Could you check a few things on this model? Use its own coordinates, in mm. A direction names the side the tool comes from. Give positions to 0.01 mm unless a question says otherwise; leave off trailing zeros. One line per item, written item: value.
Autodesk Inventor part; units mm, degrees
ref_plane "YZ Plane" through (0, 0, 0) normal (1, 0, 0) x (0, 1, 0)
ref_plane "XZ Plane" through (0, 0, 0) normal (0, 1, 0) x (-1, 0, 0)
ref_plane "XY Plane" through (0, 0, 0) normal (0, 0, 1) x (1, 0, 0)
sketch "Sketch1" plane through (0, 0, 0) normal (0, 1, 0) x (1, 0, 0)
  line L0 (300, 0) -> (-300, 0)
  line L1 (-300, 0) -> (-300, -600)
  line L2 (-300, -600) -> (300, -600)
  line L3 (300, -600) -> (300, 0)
  point P0 (0, 0)
  point P1 (0, 0)
  dimension "d0" = 600
  dimension "d1" = 600
extrude "Extrusion1" add sketch "Sketch1" along normal blind 850
sketch "Sketch2" plane through (-300, 0, 600) normal (0, 0, 1) x (-1, 0, 0)
  line L0 (-600, 0) -> (-600, -850)
  line L1 (-600, 0) -> (-570, 0)
  line L2 (-570, 0) -> (-570, -120)
  line L3 (-570, -120) -> (-600, -120)
  line L4 (-600, -120) -> (-600, 0)
  point P0 (-300, 0)
  dimension "d4" = 120
  dimension "d7" = 30
extrude "Extrusion2" cut sketch "Sketch2" against normal blind 30
move faces "Move3" translate (50, 0, 0) faces at (300, 323.3333, 190)
move faces "Move4" translate (0, 0, 50) faces at (-110, 323.3333, 600)
sketch "Sketch3" plane through (270, 120, 570) normal (0, -1, 0) x (1, 0, 0)
  line L0 (-570, 80) -> (80, 80)
  line L1 (80, 80) -> (30, 80)
  line L2 (30, 80) -> (30, 30)
  line L3 (30, 30) -> (80, 30)
  line L4 (80, 30) -> (80, 80)
  line L5 (-570, 80) -> (-570, -570)
  line L6 (-570, -570) -> (80, -570)
  point P0 (-270, -570)
  dimension "d20" = 600
  dimension "d21" = 600
extrude "Extrusion3" cut sketch "Sketch3" against normal through all
properties part number "Mobile angolo"
1) On a 3-axis mill with a long thin cutter (end or side, diameter ignored), from which of +Z, -Z, +X, -X, +Y, -Y can I reach the whole of each face in a straight line? I mean faces 1 (the face through (325, 480, 600)), 2 (the face through (311, 59, 570)), 3 (the face through (-300, 419, 320)). Say none if no direction works.
Outcome:
face 1: +Z, +X, +Y, -Y
face 2: +Z, +X, -Y
face 3: +Z, -Z, -X, +Y, -Y
2) Please list where this line runs through material, in increasing order: L1, parallel to Z at x = 321, y = 783. Write a range as from..to.
Outcome:
L1: z = 0..600
3) I'm going to push flat-ended pins straight in: pin 1 (24 mm diameter, centred on x = 326.5, y = 69.5, fed in from +Z); pin 2 (15 mm diameter, centred on y = 404, z = 615.5, fed in from +X). Where does each tip first touch, or does it pass through?
Outcome:
pin 1: stops at z = 570
pin 2: stops at x = 300
